Build history of the part. All positions in model axes, mm. A direction names the side the tool comes from. Round coordinates to 2 decimals unless told otherwise and drop trailing zeros. Order: outer loops, then holes, each group sorted by start corner. A loop starts at its lowest first (then second) coordinate and runs counter-clockwise, first axis right, second up. Notation, with made-up numbers: M -11,-27 L 32,-27 A19 ccw 32,-9 Z; hole C 8.25,35.5 d10. An arc over 180 degrees is marked long. One line per item, written item: value. Start each with the question number.
Item 1: Tool access for faces 5 (the flat face through (902, 1793.636, 25)), 6 (the flat face through (1801.537, 1795, 25)): list every direction of +Z, -Z, +X, -X, +Y, -Y with a clear straight run to the whole face (end or side of a thin tool).
Item 2: Band-saw the part on B-B, the plane x = 718.5. Write the cut outline in (y, z), then the cut area to 3 significant figures.
Item 3: Probe L1, parallel to Y at x = 776.5, z = 37.5; L2, parallel to Z at x = 342, y = 1758.5. List the from-to ranges inside material, lowest first.
Item 4: Band-saw the part on A-A, the plane z = 30.5. Write the cut outline in (x, y), then the cut area to 3 significant figures.
Item 5: Two-plate mould, pull along Y, no slides. Class faces 1 (the flat face through (876, 1797.636, 25)), 2 (the flat face through (902, 1772, 4)), 3 (the flat face through (-23.463, 1795, 25)), 4 (the flat face through (902, 1772, 46)): +Y half, -Y half, draft (parallel to the pull), parting line (faces both ways), or undercut.
```python
from build123d import *

# Parameters (mm, degrees)
F0_W     = 1825
F0_H     = 50
F0_R     = 6
F1_DEPTH = 50
F2_W     = 42
F2_H     = 42
F3_DEPTH = 1825.001


with BuildPart() as f1:
    # F0 (on Top) → F1 (new body)
    with BuildSketch(Plane.XY):
        with Locations((889.037455, 1772.636164)):
            Rectangle(F0_W, F0_H)
        with Locations((876.537455, 1772.636164)):
            Circle(F0_R, mode=Mode.SUBTRACT)
        with Locations((926.537455, 1772.636164)):
            Circle(F0_R, mode=Mode.SUBTRACT)
        with Locations((976.537455, 1772.636164)):
            Circle(F0_R, mode=Mode.SUBTRACT)
        with Locations((1026.537455, 1772.636164)):
            Circle(F0_R, mode=Mode.SUBTRACT)
        with Locations((1076.537455, 1772.636164)):
            Circle(F0_R, mode=Mode.SUBTRACT)
        with Locations((1126.537455, 1772.636164)):
            Circle(F0_R, mode=Mode.SUBTRACT)
        with Locations((1176.537455, 1772.636164)):
            Circle(F0_R, mode=Mode.SUBTRACT)
        with Locations((1326.537455, 1772.636164)):
            Circle(F0_R, mode=Mode.SUBTRACT)
        with Locations((1376.537455, 1772.636164)):
            Circle(F0_R, mode=Mode.SUBTRACT)
        with Locations((1226.537455, 1772.636164)):
            Circle(F0_R, mode=Mode.SUBTRACT)
        with Locations((1276.537455, 1772.636164)):
            Circle(F0_R, mode=Mode.SUBTRACT)
        with Locations((1426.537455, 1772.636164)):
            Circle(F0_R, mode=Mode.SUBTRACT)
        with Locations((1476.537455, 1772.636164)):
            Circle(F0_R, mode=Mode.SUBTRACT)
        with Locations((1526.537455, 1772.636164)):
            Circle(F0_R, mode=Mode.SUBTRACT)
        with Locations((1576.537455, 1772.636164)):
            Circle(F0_R, mode=Mode.SUBTRACT)
        with Locations((1626.537455, 1772.636164)):
            Circle(F0_R, mode=Mode.SUBTRACT)
        with Locations((1676.537455, 1772.636164)):
            Circle(F0_R, mode=Mode.SUBTRACT)
        with Locations((1726.537455, 1772.636164)):
            Circle(F0_R, mode=Mode.SUBTRACT)
        with Locations((1776.537455, 1772.636164)):
            Circle(F0_R, mode=Mode.SUBTRACT)
    extrude(amount=F1_DEPTH)

    # F2 (on face) → F3 (cut, through all)
    with BuildSketch(Plane.YZ.offset(1801.537455)):
        with Locations((1772.636164, 25)):
            Rectangle(F2_W, F2_H)
    extrude(amount=-F3_DEPTH, mode=Mode.SUBTRACT)


solid = f1.part
```
Output:
1. face 5: +X, -X
1. face 6: +Z, -Z, +X, +Y, -Y
2. outline: M 1747.64,0 L 1797.64,0 L 1797.64,50 L 1747.64,50 Z; hole M 1751.64,4 L 1793.64,4 L 1793.64,46 L 1751.64,46 Z
2. area: 736 mm²
3. L1: y = 1747.64 to 1751.64, 1793.64 to 1797.64
3. L2: z = 0 to 4, 46 to 50
4. outline: M -23.46,1747.64 L 1801.54,1747.64 L 1801.54,1751.64 L -23.46,1751.64 Z; M -23.46,1793.64 L 1801.54,1793.64 L 1801.54,1797.64 L -23.46,1797.64 Z
4. area: 14,600 mm²
5. face 1: +Y half
5. face 2: undercut
5. face 3: draft
5. face 4: undercut
